Could you check a few things on this model? Use its own coordinates, in mm. A direction names the side the tool comes from. Round coordinates to 2 decimals unless told otherwise and drop trailing zeros. Loops run counter-clockwise (first coordinate to the right, second up) from the corner with the lowest first, then second, coordinate; pieces in that order, holes last.
from build123d import *

# Parameters (mm, degrees)
F0_R     = 27.5
F1_DEPTH = 14
F2_SIZE  = 1


with BuildPart() as f1:
    # F0 (on Top) → F1 (new body)
    with BuildSketch(Plane.XY):
        Circle(F0_R)
        with BuildLine():
            ThreePointArc((5, 18.330303), (0, -19), (-5, 18.330303))
            Line((-5, 18.330303), (-5, 22.25))
            Line((-5, 22.25), (0, 22.25))
            Line((0, 22.25), (5, 22.25))
            Line((5, 22.25), (5, 18.330303))
        make_face(mode=Mode.SUBTRACT)
    extrude(amount=F1_DEPTH)

    # F2
    f2_edges = [f1.edges().sort_by_distance(p)[0] for p in [
        (-27.5, 0, 14),
        (-27.5, 0, 0),
    ]]
    chamfer(f2_edges, length=F2_SIZE)


solid = f1.part
Item 1: We'd pull the mould along X, two halves only. Please class faces 1 (the cylindrical face through (-5.961, -26.846, 6.916)), 2 (the flat face through (11, -17, 0)), 3 (the flat face through (-5, 20, 7)): released by +X, released by -X, zero draft, split by the parting line, or undercut.
Results list:
face 1: split by the parting line
face 2: zero draft
face 3: undercut
Item 2: If I drill on line 1 along X through (y, z) = (-0.5, 10.25); line 2 along Y through (x, z) = (0, 8.5); line 3 along Y through (x, z) = (-13, 2.25), over which ranges is the centre line in solid material (lowest first)?
Results list:
line 1: x = -27.5 to -18.99, 18.99 to 27.5
line 2: y = -27.5 to -19, 22.25 to 27.5
line 3: y = -24.23 to -13.86, 13.86 to 24.23
Item 3: If we section it at C-C, the plane z = 9: Please give me the cut outline in (x, y), then the cut area to 3 significant figures.
Results list:
outline: circle Ø55 at (0, 0); hole (-5, 18.33) arc R19 ccw (long way) to (5, 18.33) - (5, 22.25) - (-5, 22.25) - close
area: 1,210 mm2
Item 4: Will these pins go through, and if not, where does the flat tip stop? pin 1 (3 mm diameter, centred on x = -13, z = 6.5, fed in from -Y); pin 2 (3 mm diameter, centred on y = 20.5, z = 10, fed in from -X); pin 3 (6 mm diameter, centred on y = 8, z = 8.5, fed in from -X).
Results list:
pin 1: stops at y = -24.98
pin 2: stops at x = -19.88
pin 3: stops at x = -27.04
Item 5: If we section it at B-B, the plane y = 0: Please give me the cut outline in (x, z), then the cut area to 3 significant figures.
Results list:
outline: (-27.5, 1) - (-26.5, 0) - (-19, 0) - (-19, 14) - (-26.5, 14) - (-27.5, 13) - close; (19, 0) - (26.5, 0) - (27.5, 1) - (27.5, 13) - (26.5, 14) - (19, 14) - close
area: 236 mm2
Item 6: For faces 4 (the flat face through (5, 20, 7)), 5 (the flat face through (11, -17, 14)), which set-ups out of +Z, -Z, +X, -X, +Y, -Y let a thin tool reach every point of the face, with its end or its side?
Results list:
face 4: +Z, -Z
face 5: +Z, +X, -X, +Y, -Y
Item 7: If we section it at A-A, the plane x = 0: Please give me the cut outline in (y, z).
Results list:
outline: (-27.5, 1) - (-26.5, 0) - (-19, 0) - (-19, 14) - (-26.5, 14) - (-27.5, 13) - close; (22.25, 0) - (26.5, 0) - (27.5, 1) - (27.5, 13) - (26.5, 14) - (22.25, 14) - close
